Autodesk Inventor part; units mm, degrees
ref_plane "YZ Plane" through (0, 0, 0) normal (1, 0, 0) x (0, 1, 0)
ref_plane "XZ Plane" through (0, 0, 0) normal (0, 1, 0) x (-1, 0, 0)
ref_plane "XY Plane" through (0, 0, 0) normal (0, 0, 1) x (1, 0, 0)
sketch "Esquisse1" plane through (0, 0, 0) normal (0, 1, 0) x (-1, 0, 0)
  line L0 (-27.75, 33) -> (27.75, 33)
  line L1 (27.75, 33) -> (27.75, -33)
  line L2 (27.75, -33) -> (-27.75, -33)
  line L3 (-27.75, -33) -> (-27.75, 33)
  line L4 (-27.75, 33) -> (27.75, -33) construction
  line L5 (27.75, 33) -> (-27.75, -33) construction
  point P0 (0, 0)
  dimension "d0" = 66
  dimension "d1" = 55.5
extrude "Extrusion1" add sketch "Esquisse1" along normal blind 35.5
sketch "Esquisse2" plane through (27.75, 0, 33) normal (1, 0, 0) x (0, 0, -1)
  circle A0 centre (40, 26.75) radius 1.5
  circle A1 centre (40, 8.75) radius 1.5
  line L0 (66, 0) -> (66, 35.5)
  circle A2 centre (25, 8.75) radius 1.5
  circle A3 centre (25, 26.75) radius 1.5
  circle A4 centre (10, 8.75) radius 1.5
  circle A5 centre (10, 26.75) radius 1.5
  line L1 (66, 0) -> (0, 0)
  line L2 (40, 8.75) -> (40, 26.75)
  line L3 (40, 26.75) -> (25, 26.75)
  line L4 (25, 26.75) -> (10, 26.75)
  line L5 (10, 26.75) -> (10, 8.75)
  line L6 (10, 8.75) -> (25, 8.75)
  line L7 (25, 8.75) -> (25, 26.75)
  line L8 (25, 8.75) -> (40, 8.75)
  line L9 (40, 26.75) -> (66, 26.75)
  line L10 (40, 8.75) -> (66, 8.75)
  circle A6 centre (51, 17.75) radius 8
  circle A7 centre (41, 17.75) radius 0.75
  line L11 (0, 0) -> (0, 35.5)
  line L12 (0, 17.75) -> (66, 17.75)
  circle A8 centre (56, 9.0897) radius 0.75
  circle A9 centre (56, 26.4103) radius 0.75
  point P0 (33, 0)
  point P1 (40, 17.75)
  point P2 (10, 17.75)
  dimension "d4" = 18
  dimension "d5" = 3
  dimension "d22" = 16
  dimension "d27" = 1.5
  dimension "d61" = 10
  dimension "d62" = 15
  dimension "d63" = 15
  dimension "d64" = 51
  dimension "d65" = 10
  dimension "d68" = 360
hole "Perçage1" at (27.75, 26.75, 23) at (27.75, 26.75, 8) at (27.75, 26.75, -7) at (27.75, 8.75, -7) at (27.75, 8.75, 8) at (27.75, 8.75, 23) direction (-1, 0, 0) diameter 3 depth 5 tip angle 118
mirror "Mise en miroir1" about plane through (0, 0, 0) normal (1, 0, 0) of "Perçage1"
extrude "Extrusion2" add sketch "Esquisse2" along normal blind 2 contours A9 L9 | L9 A9 | L12 A7 | A7 L12 | A8 L10 | L10 A8
extrude "Extrusion3" add sketch "Esquisse2" along normal blind 15 contours L12 A6 | A6 L12
sketch "Esquisse4" plane through (-27.75, 0, 33) normal (0, 0, 1) x (1, 0, 0)
  circle A0 centre (37.4, 17.75) radius 15
  line L0 (0, 0) -> (55.5, 0)
  circle A1 centre (51.7, 31.75) radius 1.5
  circle A2 centre (51.7, 3.75) radius 1.5
  line L1 (55.5, 0) -> (55.5, 35.5)
  line L2 (55.5, 3.75) -> (51.7, 3.75)
  line L3 (51.7, 3.75) -> (51.7, 31.75)
  line L4 (51.7, 31.75) -> (55.5, 31.75)
  circle A3 centre (16.7, 31.75) radius 1.5
  circle A4 centre (16.7, 3.75) radius 1.5
  circle A5 centre (3.7, 31.75) radius 1.5
  circle A6 centre (3.7, 3.75) radius 1.5
  line L5 (16.7, 31.75) -> (16.7, 3.75)
  line L6 (16.7, 3.75) -> (3.7, 3.75)
  line L7 (3.7, 3.75) -> (3.7, 31.75)
  line L8 (3.7, 31.75) -> (16.7, 31.75)
  line L9 (51.7, 31.75) -> (16.7, 31.75)
  line L10 (16.7, 3.75) -> (51.7, 3.75)
  circle A7 centre (37.4, 5.75) radius 2
  circle A8 centre (37.4, 17.75) radius 12
  circle A9 centre (49.4, 17.75) radius 2
  circle A10 centre (37.4, 29.75) radius 2
  circle A11 centre (25.4, 17.75) radius 2
  line L11 (0, 0) -> (0, 35.5)
  point P0 (27.75, 0)
  point P1 (51.7, 17.75)
  dimension "d40" = 24
  dimension "d32" = 17.75
  dimension "d33" = 30
  dimension "d34" = 28
  dimension "d35" = 3
  dimension "d36" = 3.8
  dimension "d38" = 35
  dimension "d39" = 13
  dimension "d41" = 4
  dimension "d44" = 360
  dimension "d48" = 17.75
  dimension "d59" = 37.4
  dimension "d60" = 18.1
  dimension "d70" = 3.7
extrude "Extrusion4" add sketch "Esquisse4" along normal blind 5.1 contours A0 L3 | L3 A0 L10 A7 A8 A9 A10 L9 | L9 A0 | A0 L10 | L9 A10 A8 A11 A7 L10 A0 | A10 A8 A9 A7 A11
hole "Perçage2" at (23.95, 31.75, 33) at (23.95, 3.75, 33) at (-11.05, 3.75, 33) at (-24.05, 3.75, 33) at (-24.05, 31.75, 33) at (-11.05, 31.75, 33) direction (0, 0, -1) diameter 3 depth 6 tip angle 118
sketch "Esquisse5" plane through (27.75, 0, -33) normal (0, 0, -1) x (-1, 0, 0)
  circle A0 centre (18.1, 17.75) radius 15
  circle A1 centre (18.1, 17.75) radius 15
  circle A2 centre (6.1, 17.75) radius 2
  circle A3 centre (6.1, 17.75) radius 2
  circle A4 centre (18.1, 29.75) radius 2
  circle A5 centre (18.1, 29.75) radius 2
  circle A6 centre (30.1, 17.75) radius 2
  circle A7 centre (30.1, 17.75) radius 2
  circle A8 centre (18.1, 5.75) radius 2
  circle A9 centre (18.1, 5.75) radius 2
  point P0 (27.75, 0)
  dimension "d56" = 30
extrude "Extrusion5" add sketch "Esquisse5" along normal blind 8
properties part number "Servo_moteur_rovmaker"
Geometry: final body of the model. Coordinates: model frame, mm. A direction names the side the tool comes from. Coordinates: 2 decimals unless noted, no trailing zeros. Order: outer loops, then holes, each group sorted by start corner. A loop starts at its lowest first (then second) coordinate and runs counter-clockwise, first axis right, second up. Notation, with made-up numbers: (-8, 78) -> (8, 78) arc R19 cw to (8, 108) -> close; hole circle Ø11 at (42.25, -14.5). An arc over 180 degrees is marked (long way). Write each question's results on one line, items separated by ' | '. Start each with the question number.
1) Cut plane D-D, the plane z = 1.5. Output: boundary loops of the cut face in (x, y).
2) First-contact query: pin 1 (2.5 mm diameter, centred on x = 21.65, y = 17.75, fed in from +Z); pin 2 (2.5 mm diameter, centred on x = -11.05, y = 3.75, fed in from +Z); pin 3 (3 mm diameter, centred on x = -2, y = 18, fed in from -Z). Flat tips, straight axial feed; report the tip coordinate or a pass-through.
3) Mould query, pull axis X, two halves, no side actions, for faces 1 (the cylindrical face through (9.2, 31.7, 35.5)), 2 (the cylindrical face through (1.59, 5.1, -36.94)), 3 (the cylindrical face through (-25.22, 7.84, -5.81)). Classes: released by +X, released by -X, zero draft, split by the parting line, or undercut.
4) Cut plane B-B, the plane z = -18. Output: boundary loops of the cut face in (x, y).
5) Material intervals for line 1 along Y through (x, z) = (-26, 8); line 2 along Y through (x, z) = (-24, 28); line 3 along X through (y, z) = (17.75, 35.1), sorted ascending.
6) Cut plane A-A, the plane x = 9.65. Output: boundary loops of the cut face in (y, z), and give its area (3 significant figures).
7) Cut plane C-C, the plane x = -2.35. Output: boundary loops of the cut face in (y, z).
8) Set-up query: faces 4 (the cylindrical face through (25.22, 9.66, 24.19)), 5 (the flat face through (9, 18, 38.1)), 6 (the cylindrical face through (-9.7, 3.1, 30)), 7 (the flat face through (10, 30, -33)). Return all of +Z, -Z, +X, -X, +Y, -Y with unobstructed straight access to the full face (end or side cutting, diameter ignored); none if empty.
Checks:
1) outline: (-27.75, 0) -> (27.75, 0) -> (27.75, 35.5) -> (-27.75, 35.5) -> close
2) pin 1: z = 33 | pin 2: z = 26.85 | pin 3: z = -33
3) face 1: undercut | face 2: split by the parting line | face 3: zero draft
4) outline: (-27.75, 0) -> (27.75, 0) -> (27.75, 9.75) -> (42.75, 9.75) -> (42.75, 25.75) -> (27.75, 25.75) -> (27.75, 35.5) -> (-27.75, 35.5) -> close
5) line 1: 0 to 7.25, 10.25 to 25.25, 28.25 to 35.5 | line 2: 0 to 2.25, 5.25 to 30.25, 33.25 to 35.5 | line 3: -5.35 to -4.35, -0.35 to 19.65, 23.65 to 24.65
6) outline: (0, -33) -> (2.75, -33) -> (2.75, -41) -> (3.75, -41) -> (3.75, -33) -> (7.75, -33) -> (7.75, -41) -> (27.75, -41) -> (27.75, -33) -> (31.75, -33) -> (31.75, -41) -> (32.75, -41) -> (32.75, -33) -> (35.5, -33) -> (35.5, 33) -> (32.75, 33) -> (32.75, 38.1) -> (31.75, 38.1) -> (31.75, 33) -> (27.75, 33) -> (27.75, 38.1) -> (7.75, 38.1) -> (7.75, 33) -> (3.75, 33) -> (3.75, 38.1) -> (2.75, 38.1) -> (2.75, 33) -> (0, 33) -> close | area: 2,630 mm^2
7) outline: (0, -33) -> (8.75, -33) -> (8.75, -41) -> (15.75, -41) -> (15.75, -33) -> (19.75, -33) -> (19.75, -41) -> (26.75, -41) -> (26.75, -33) -> (35.5, -33) -> (35.5, 33) -> (26.75, 33) -> (26.75, 38.1) -> (19.75, 38.1) -> (19.75, 33) -> (15.75, 33) -> (15.75, 38.1) -> (8.75, 38.1) -> (8.75, 33) -> (0, 33) -> close
8) face 4: +X | face 5: +Z, +X, -X, +Y, -Y | face 6: +Z | face 7: -Z
